from build123d import *

# Parameters (mm, degrees)
F0_R     = 1.75
F1_DEPTH = 4
F3_R     = 4.245
F4_DEPTH = 23.101011


with BuildPart() as f1:
    # F0 (on Front) → F1 (new body)
    with BuildSketch(Plane.XZ):
        Polygon((-15, 30), (-15, 0), (-15, -30), (0, -30), (15, -30), (15, 0), (15, 30), (0, 30), align=None)
        with Locations((0, -11.75)):
            Circle(F0_R, mode=Mode.SUBTRACT)
        with Locations((0, 11.75)):
            Circle(F0_R, mode=Mode.SUBTRACT)
    extrude(amount=F1_DEPTH)

    # F3 (on face) → F4 (join)
    with BuildSketch(Plane.XZ.offset(4)):
        Circle(F3_R)
    extrude(amount=F4_DEPTH)


solid = f1.part
For this review, take the finished solid that the model builds, in its own axes (mm). Give positions to 0.01 mm unless a question says otherwise; leave off trailing zeros. Loops run counter-clockwise (first coordinate to the right, second up) from the corner with the lowest first, then second, coordinate; pieces in that order, holes last.
Item 1: Take a section at B-B, the plane x = 0. State the section outline as (y, z) points (3 decimals).
Item 2: For line 1 along Z through (x, y) = (0, -0.85); line 2 along Y through (x, z) = (-5.75, 23); line 3 along Z through (x, y) = (0.5, -24), list the stretches that pass through material, from the lowest coordinate up.
Item 3: Draft analysis for pull direction X (two halves, no side actions). For faces 1 (the flat face through (15, -2, 0)), 2 (the cylindrical face through (-0.228, -1.972, 13.485)), 3 (the cylindrical face through (2.28, -15.39, 3.58)), 4 (the flat face through (0, -4, 7)), state which applies: +X half, -X half, draft (parallel to the pull), parting line (faces both ways), or undercut.
Item 4: Take a section at D-D, the plane y = -21. State the section outline as (x, z) points (3 decimals), and give its area (3 significant figures).
Item 5: Take a section at C-C, the plane z = 0. State the section outline as (x, y) points (3 decimals), and give its area (3 significant figures).
Item 6: Take a section at A-A, the plane z = -11.75. State the section outline as (x, y) points, and give its area (3 significant figures).
Item 7: Insertion check: pin 1 (10 mm diameter, centred on x = -9.5, y = -12.5, fed in from +Z); pin 2 (4 mm diameter, centred on x = 2, y = -12.5, fed in from +Z) (3 decimals); pin 3 (10 mm diameter, centred on y = -6.5, z = 8.5, fed in from -X); pin 4 (5 mm diameter, centred on x = 0.5, y = -16.5, fed in from -Z) (3 decimals). Each pin has a flat end and moves straight along its axis. Give the tip position at first contact, or say it passes through.
Calculated:
1. outline: (-27.101, -4.245) - (-4, -4.245) - (-4, -10) - (0, -10) - (0, 10) - (-4, 10) - (-4, 4.245) - (-27.101, 4.245) - close; (-4, -30) - (0, -30) - (0, -13.5) - (-4, -13.5) - close; (-4, 13.5) - (0, 13.5) - (0, 30) - (-4, 30) - close
2. line 1: z = -30 to -13.5, -10 to 10, 13.5 to 30
2. line 2: y = -4 to 0
2. line 3: z = -4.22 to 4.22
3. face 1: +X half
3. face 2: undercut
3. face 3: parting line
3. face 4: draft
4. outline: circle Ø8.49 at (0, 0)
4. area: 56.6 mm2
5. outline: (-15, -4) - (-4.245, -4) - (-4.245, -27.101) - (4.245, -27.101) - (4.245, -4) - (15, -4) - (15, 0) - (-15, 0) - close
5. area: 316 mm2
6. outline: (-15, -4) - (-1.75, -4) - (-1.75, 0) - (-15, 0) - close; (1.75, -4) - (15, -4) - (15, 0) - (1.75, 0) - close
6. area: 106 mm2
7. pin 1: passes through
7. pin 2: stops at z = 4.245
7. pin 3: stops at x = -15
7. pin 4: stops at z = -4.245
